Source: CAD feature listing. Evaluate the final solid. Frame: model axes, mm. A direction names the side the tool comes from. Give positions to 0.01 mm unless a question says otherwise; leave off trailing zeros. Write each loop counter-clockwise with the first axis right and the second up, starting at its lowest first coordinate (ties: lowest second). Pieces come first, ordered by that corner, then holes. Notation, with made-up numbers: M 6,-30 L 47,-30 A3 ccw 47,-26 Z; hole C 11.5,49 d5. An arc over 180 degrees is marked long. Return JSON: item names as keys, results as strings.
Autodesk Inventor part; units mm, degrees
ref_plane "Work Plane1" through (0, -1.5, 0) normal (0, 1, 0) x (-1, 0, 0)
ref_plane "YZ Plane" through (0, 0, 0) normal (1, 0, 0) x (0, 1, 0)
ref_plane "XY Plane" through (0, 0, 0) normal (0, 0, 1) x (1, 0, 0)
sketch "Sketch1" plane through (0, 0, 0) normal (0, 1, 0) x (-1, 0, 0)
  line L0 (5.2, -8.1) -> (-5.2, -8.1)
  line L1 (-5.2, -8.1) -> (-5.2, 8.1)
  line L2 (-5.2, 8.1) -> (5.2, 8.1)
  line L3 (5.2, 8.1) -> (5.2, -8.1)
  line L4 (5.2, -8.1) -> (-5.2, 8.1) construction
  line L5 (-5.2, -8.1) -> (5.2, 8.1) construction
  point P0 (0, 0)
  dimension "d0" = 16.2
  dimension "d1" = 10.4
extrude "Extrusion1" add sketch "Sketch1" along normal blind 0.3 draft -5 and the other way blind 2.9 draft -5
sketch "Sketch2" plane through (0, -2.9, 0) normal (0, -1, 0) x (1, 0, 0)
  line L0 (-4.9463, -7.8463) -> (-4.9463, 7.8463)
  line L1 (4.9463, -7.8463) -> (-4.9463, -7.8463)
  line L2 (4.9463, 7.8463) -> (4.9463, -7.8463)
  line L3 (-4.9463, 7.8463) -> (4.9463, 7.8463)
  circle A0 centre (0, 4.9) radius 1.6
  line L4 (5.2, 8.1) -> (-5.2, 8.1)
  point P0 (0, 0)
  dimension "d6" = 3.2
  dimension "d7" = 3.2
extrude "Extrusion2" cut sketch "Sketch2" against normal through all contours A0
sketch "Sketch3" plane through (0, -2.9, 0) normal (0, -1, 0) x (1, 0, 0)
  line L0 (-4.9463, -7.8463) -> (-4.9463, 7.8463)
  line L1 (-5.2, 8.1) -> (-4.9463, 7.8463)
  line L2 (-5.2, 8.1) -> (-5.2, -8.1)
  line L3 (-5.2, -8.1) -> (-4.9463, -7.8463)
  circle A0 centre (0, 4.9) radius 1.6
  line L4 (-4.9463, -7.8463) -> (-4.9463, 7.8463)
  line L5 (4.9463, -7.8463) -> (-4.9463, -7.8463)
  line L6 (4.9463, 7.8463) -> (4.9463, -7.8463)
  line L7 (-4.9463, 7.8463) -> (4.9463, 7.8463)
  line L8 (4.9463, 7.8463) -> (4.9463, -7.8463)
  line L9 (5.2, -8.1) -> (4.9463, -7.8463)
  line L10 (5.2, -8.1) -> (5.2, 8.1)
  line L11 (5.2, 8.1) -> (4.9463, 7.8463)
  line L12 (-5.2, 8.1) -> (-5.2, -8.1)
  arc A1 (-5.2, 3.6) -> (-5.2, 6.2) centre (-5.2, 4.9) ccw
  line L13 (5.2, -8.1) -> (5.2, 8.1)
  arc A2 (5.2, 6.2) -> (5.2, 3.6) centre (5.2, 4.9) ccw
  point P0 (0, 0)
  dimension "d10" = 1.3
extrude "Extrusion3" cut sketch "Sketch3" against normal up to surface (2.9 mm away) contours A1 L2 L0 | L0 A1 | A2 L6 | L6 A2 L10
ref_plane "Work Plane1" through (0, -1.5, 0) normal (0, 1, 0) x (-1, 0, 0)
sketch "Sketch4" plane through (0, -1.5, 0) normal (0, 1, 0) x (-1, 0, 0)
  line L0 (-4.9463, -7.8463) -> (4.9463, -7.8463)
  line L1 (5.2, -8.1) -> (4.9463, -7.8463)
  line L2 (5.2, -8.1) -> (-5.2, -8.1)
  line L3 (-5.2, -8.1) -> (-4.9463, -7.8463)
  line L4 (3.19, -7.8463) -> (3.19, -11.563)
  line L5 (5.2, -8.1) -> (-5.2, -8.1)
  line L6 (3.19, -11.563) -> (3.04, -11.563)
  arc A0 (3.04, -11.563) -> (2.94, -11.663) centre (3.04, -11.663) ccw
  line L7 (2.94, -11.663) -> (2.94, -13.663)
  line L8 (2.94, -13.663) -> (2.14, -13.663)
  line L9 (2.14, -13.663) -> (2.14, -11.663)
  arc A1 (2.14, -11.663) -> (2.04, -11.563) centre (2.04, -11.663) ccw
  line L10 (2.04, -11.563) -> (1.89, -11.563)
  line L11 (1.89, -7.8463) -> (1.89, -11.563)
  circle A2 centre (0, 4.9) radius 1.6
  dimension "d21" = 0.8
  dimension "d22" = 1.3
  dimension "d23" = 0.1
  dimension "d24" = 16.463
  dimension "d25" = 1.89
  dimension "d26" = 2.1
extrude "Extrusion4" add sketch "Sketch4" against normal blind 0.6 contours L0 L4 L2 L11 | L2 L4 L6 A0 L7 L8 L9 A1 L10 L11
mirror "Mirror1" about plane through (0, 0, 0) normal (1, 0, 0) of "Extrusion4"
sketch "Sketch5" plane through (0, 0.3, 0) normal (0, 1, 0) x (1, 0, 0)
  circle A0 centre (0, -4.9) radius 1.6
  line L0 (5.1738, 8.0738) -> (5.1738, -8.0738)
  line L1 (-5.1738, 8.0738) -> (5.1738, 8.0738)
  line L2 (-5.1738, -8.0738) -> (-5.1738, 8.0738)
  line L3 (5.1738, -8.0738) -> (-5.1738, -8.0738)
  line L4 (4.25, -2.237) -> (-4.25, -2.237)
  line L5 (-4.25, -2.237) -> (-4.25, 7.163)
  line L6 (-4.25, 7.163) -> (4.25, 7.163)
  line L7 (4.25, 7.163) -> (4.25, -2.237)
  point P0 (0, 0)
  point P1 (0, -2.237)
  dimension "d34" = 8.5
  dimension "d35" = 9.4
  dimension "d36" = 2.663
split_face "Split1"
properties part number "Resistor_TH-TO220" material "ABS Plastic"
1) Cut plane B-B, the plane z = 4.9. Return the cut outline in (x, y), then the cut area to 3 significant figures.
Numbers:
{"outline": "M -5.2,0 L -3.9,0 L -3.9,-2.9 L -1.6,-2.9 L -1.6,0.3 L -5.17,0.3 Z; M 1.6,-2.9 L 3.9,-2.9 L 3.9,0 L 5.2,0 L 5.17,0.3 L 1.6,0.3 Z", "area": "15.5 mm²"}
2) Line query: line 1 (X direction, y = -1.6, z = 5.25); line 2 (Z direction, x = 0, y = -1.3); line 3 (Z direction, x = -4.5, y = -1.9). Output: solid intervals per line, ascending. Write a range as [from, to].
Numbers:
{"line 1": "x = [-3.95, -1.56], [1.56, 3.95]", "line 2": "z = [-7.99, 3.3], [6.5, 7.99]", "line 3": "z = [-7.93, 3.8], [6, 7.93]"}
3) Cut plane D-D, the plane z = -10.5. Return the cut outline in (x, y), then the cut area to 3 significant figures.
Numbers:
{"outline": "M -3.19,-2.1 L -1.89,-2.1 L -1.89,-1.5 L -3.19,-1.5 Z; M 1.89,-2.1 L 3.19,-2.1 L 3.19,-1.5 L 1.89,-1.5 Z", "area": "1.56 mm²"}
4) Contact query for flat-ended pins moving along their axis: pin 1 Ø1 at (y, z) = (-2, -5.5) entering from +X; pin 2 Ø1.4 at (x, z) = (5, 5) entering from -Y; pin 3 Ø0.5 at (y, z) = (-2, -9.5) entering from -X; pin 4 Ø1.9 at (x, z) = (0, 4.9) entering from -Y. Output: stop coordinate, or through.
Numbers:
{"pin 1": "stops at x = 5.07", "pin 2": "stops at y = 0", "pin 3": "stops at x = -3.19", "pin 4": "passes through"}
5) Set-up query: faces 4 (the face through (3, -2.1, -10)), 5 (the face through (3.9, -1.5, 4.9)), 6 (the face through (-3.9, -1.5, 4.9)). Return all of +Z, -Z, +X, -X, +Y, -Y with unobstructed straight access to the full face (end or side cutting, diameter ignored); none if empty.
Numbers:
{"face 4": "-Z, +X, -X, -Y", "face 5": "+X, -Y", "face 6": "-X, -Y"}
6) Cut plane A-A, the plane x = 0. Return the cut outline in (y, z), then the cut area to 3 significant figures.
Numbers:
{"outline": "M -2.9,-7.85 L 0,-8.1 L 0.3,-8.07 L 0.3,3.3 L -2.9,3.3 Z; M -2.9,6.5 L 0.3,6.5 L 0.3,8.07 L 0,8.1 L -2.9,7.85 Z", "area": "40.9 mm²"}
7) Cut plane C-C, the plane y = -1.3. Return the cut outline in (x, z), then the cut area to 3 significant figures.
Numbers:
{"outline": "M -5.09,-7.99 L 5.09,-7.99 L 5.09,3.6 A1.3 cw 5.09,6.2 L 5.09,7.99 L -5.09,7.99 L -5.09,6.2 A1.3 cw -5.09,3.6 Z; hole C 0,4.9 d3.2", "area": "150 mm²"}
8) Draft query along Z for faces 1 (the face through (0.073, -1.43, 7.975)), 2 (the face through (5, 0, 5)), 3 (the face through (5.075, -1.43, 7.124)). Return one class per face: released by +Z, released by -Z, zero draft, split by the parting line, or undercut.
Numbers:
{"face 1": "released by +Z", "face 2": "undercut", "face 3": "zero draft"}
